Verification items for this drawing (mm, ordinates from the low corner). Round coordinates to 2 decimals unless told otherwise and drop trailing zeros. Loops run counter-clockwise (first coordinate to the right, second up) from the corner with the lowest first, then second, coordinate; pieces in that order, holes last. Notation, with made-up numbers: M 76.5,69 L 126.5,69 A4 cw 126.5,73 Z; hole C 57,44 d7. An arc over 180 degrees is marked long. Write item = value, one per line.
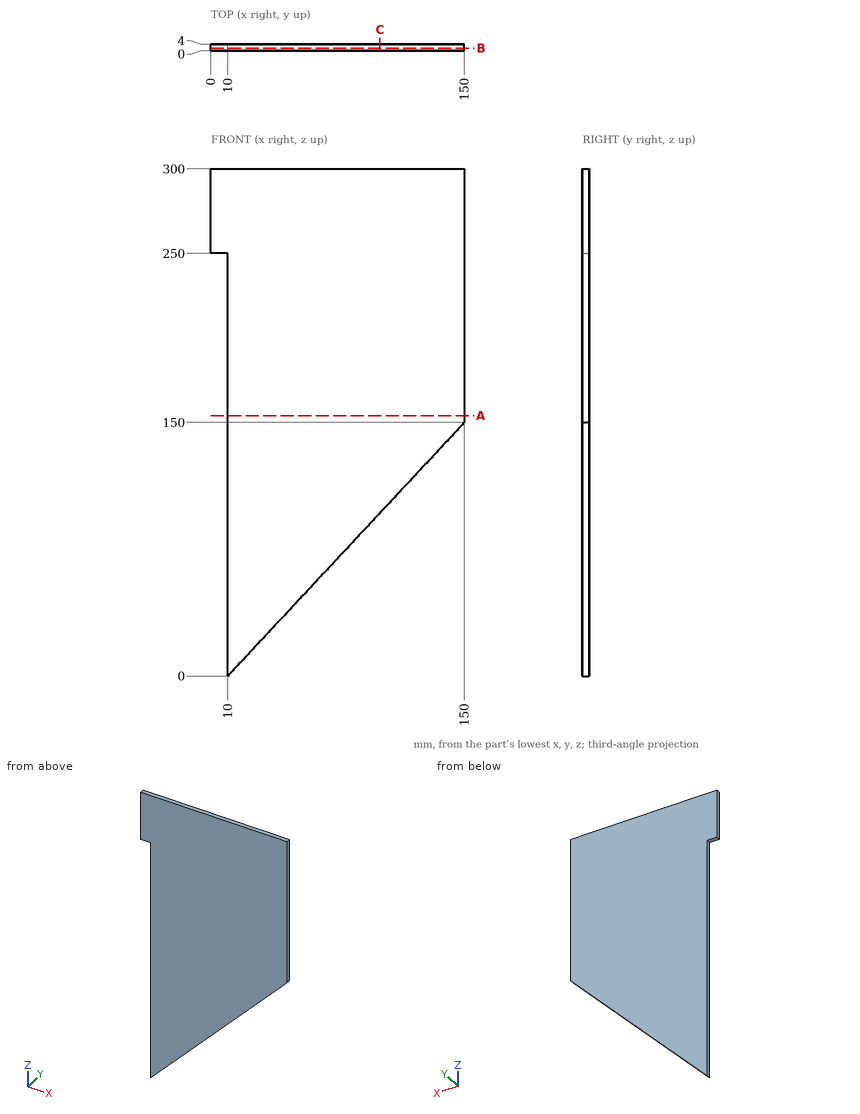
(1) Material ranges on line 1 along X through (y, z) = (2.75, 189); line 2 along Z through (x, y) = (9.5, 1.65); line 3 along X through (y, z) = (2.35, 43), recorded low to high. Write a range as from..to.
Result set:
line_1 = 10..150
line_2 = 250..300
line_3 = 10..50.13
(2) Sectioned sample at B-B on y = 1.55. Record the cut outline in (x, z).
Result set:
outline = M 0,250 L 10,250 L 10,0 L 150,150 L 150,300 L 0,300 Z
(3) Sectioned sample at A-A on z = 154. Record the cut outline in (x, y).
Result set:
outline = M 10,0 L 150,0 L 150,4 L 10,4 Z
(4) Sectioned sample at C-C on x = 100. Record the cut outline in (y, z).
Result set:
outline = M 0,96.43 L 4,96.43 L 4,300 L 0,300 Z
(5) Depth check by flat-ended pin: pin 1 Ø1.2 at (x, y) = (3.5, 1.5) entering from -Z; pin 2 Ø1 at (y, z) = (2, 71.5) entering from -X; pin 3 Ø1.5 at (y, z) = (1.5, 96) entering from +X. Enter the tip coordinate at first touch or a pass-through.
Result set:
pin_1 = 250
pin_2 = 10
pin_3 = 100.3
